Geometry check sheet. Reference: the model listing, model coordinates, mm. A direction names the side the tool comes from. Give positions to 0.01 mm unless a question says otherwise; leave off trailing zeros. Loops run counter-clockwise (first coordinate to the right, second up) from the corner with the lowest first, then second, coordinate; pieces in that order, holes last. Notation, with made-up numbers: (53, 74) - (63, 74) arc R24 cw to (63, 89) - close; hole circle Ø9 at (75.5, 1). An arc over 180 degrees is marked (long way). Use a Markdown table: item, result. Add a question column.
1. Cross-section at A-A on y = 0. Enter the section's corners in (x, z), and give its area (3 significant figures).
2. Material ranges on L1, parallel to Z at x = -2, y = -1; L2, parallel to Z at x = 3, y = 1.75; L3, parallel to X at y = 1.75, z = 0.5, recorded low to high.
3. Cross-section at D-D on z = -3. Enter the section's corners in (x, y).
4. Depth check by flat-ended pin: P1, Ø3, axis at x = 1.5, z = 9, coming from the +Y side; P2, Ø1.5, axis at x = -1.5, z = 0, coming from the -Y side; P3, Ø3, axis at x = 1, z = 1, coming from the -Y side; P4, Ø2, axis at y = -3, z = 5, coming from the +X side. Enter the tip coordinate at first touch or a pass-through.
5. Cross-section at C-C on z = 3. Enter the section's corners in (x, y), and give its area (3 significant figures).
6. Set-up check for faces 1 (the cylindrical face through (-2.579, -1.978, 6.684)), 2 (the cylindrical face through (-0.867, -3.905, 0.986)), 3 (the cylindrical face through (0, -2, -3)): record each of +Z, -Z, +X, -X, +Y, -Y from which the full face is reachable in a straight line by a thin tool's end or side.
from build123d import *

# Parameters (mm, degrees)
F0_R     = 4
F0_R_2   = 2
F1_DEPTH = 2
F2_R     = 3.25
F3_DEPTH = 10
F4_DEPTH = 7
F5_R     = 0.5


with BuildPart() as f1:
    # F0 (on Top) → F1 (new body)
    with BuildSketch(Plane.XY):
        Circle(F0_R)
        Circle(F0_R_2, mode=Mode.SUBTRACT)
        Circle(F0_R_2)
    extrude(amount=F1_DEPTH)

    # F2 (on face) → F3 (join)
    with BuildSketch(Plane.XY.offset(2)):
        Circle(F2_R)
    extrude(amount=F3_DEPTH)

    # F0 (on Top) → F4 (join)
    with BuildSketch(Plane.XY):
        Circle(F0_R_2)
    extrude(amount=-F4_DEPTH)

    # F5
    f5_edges = [f1.edges().sort_by_distance(p)[0] for p in [
        (-3.25, 0, 12),
    ]]
    fillet(f5_edges, radius=F5_R)


solid = f1.part
Values found:
| question | item | result |
|---|---|---|
| 1 | outline | (-4, 0) - (-2, 0) - (-2, -7) - (2, -7) - (2, 0) - (4, 0) - (4, 2) - (3.25, 2) - (3.25, 11.5) arc R0.5 ccw to (2.75, 12) - (-2.75, 12) arc R0.5 ccw to (-3.25, 11.5) - (-3.25, 2) - (-4, 2) - close |
| 1 | area | 109 mm2 |
| 2 | L1 | z = 0 to 12 |
| 2 | L2 | z = 0 to 2 |
| 2 | L3 | x = -3.6 to 3.6 |
| 3 | outline | circle Ø4 at (0, 0) |
| 4 | P1 | stops at y = 3.25 |
| 4 | P2 | stops at y = -3.93 |
| 4 | P3 | stops at y = -4 |
| 4 | P4 | stops at x = 2.56 |
| 5 | outline | circle Ø6.5 at (0, 0) |
| 5 | area | 33.2 mm2 |
| 6 | face 1 | +Z |
| 6 | face 2 | +Z, -Z |
| 6 | face 3 | -Z |
